Geometry: final body of the model. Coordinates: model frame, mm. A direction names the side the tool comes from. Round coordinates to 2 decimals unless told otherwise and drop trailing zeros. Loops run counter-clockwise (first coordinate to the right, second up) from the corner with the lowest first, then second, coordinate; pieces in that order, holes last. Notation, with made-up numbers: (61, 38.5) - (115, 38.5) arc R28 ccw to (115, 68.5) - close; hole circle Ø1 at (-38, 11). An arc over 180 degrees is marked (long way). Answer as CSV lines item,"result".
from build123d import *

# Parameters (mm, degrees)
BOSS_EXTRUDE1_DEPTH     = 10
SKETCH2_W               = 10
SKETCH2_H               = 2.000056303
BOSS_EXTRUDE2_DEPTH     = 5
CUT_EXTRUDE3_DEPTH      = 11
BOSS_EXTRUDE7_DEPTH     = 10
SKETCH10_R              = 42.5
CUT_EXTRUDE5_DEPTH      = 2
CUT_EXTRUDE5_DEPTH_BACK = 2


with BuildPart() as part:
    # Sketch1 → Boss-Extrude1 (new body)
    with BuildSketch(Plane.XY):
        with BuildLine():
            Line((-0.275264024, 0.618336289), (-0.275264024, 20.618336289))
            ThreePointArc((-0.275264024, 20.618336289), (-1.471073772, 23.494405264), (-4.353490365, 24.674832426))
            Line((-4.353490365, 24.674832426), (-4.353490365, 22.674776123))
            ThreePointArc((-4.353490365, 22.674776123), (-2.885297366, 22.080181828), (-2.275264024, 20.618336289))
            Line((-2.275264024, 20.618336289), (-2.275264024, 0.618336289))
            Line((-2.275264024, 0.618336289), (-1.040586258, -1.454212886))
            Line((-1.040586258, -1.454212886), (0.959413742, -1.454212886))
            Line((0.959413742, -1.454212886), (-0.275264024, 0.618336289))
        make_face()
    extrude(amount=BOSS_EXTRUDE1_DEPTH)

    # Sketch2 → Boss-Extrude2 (add)
    with BuildSketch(Plane.ZY.offset(4.353490365)):
        with Locations((5, 23.674804275)):
            Rectangle(SKETCH2_W, SKETCH2_H)
    extrude(amount=BOSS_EXTRUDE2_DEPTH)

    # Sketch7 → Cut-Extrude3 (cut, through all)
    with BuildSketch(Plane.XY.offset(10)):
        with BuildLine():
            Line((-9.353490365, 24.674832426), (-8.891740984, 22.674776123))
            ThreePointArc((-8.891740984, 22.674776123), (-9.122615674, 22.648471274), (-9.353490365, 22.674776123))
            Line((-9.353490365, 22.674776123), (-9.353490365, 24.674832426))
        make_face()
    extrude(amount=-CUT_EXTRUDE3_DEPTH, mode=Mode.SUBTRACT)

    # Sketch8 → Boss-Extrude7 (add, through all)
    with BuildSketch(Plane.XY.offset(10)):
        Polygon((-9.122615674, 23.674804274), (-50.533343428, 14.114384465), (-50.555838533, 14.211821471), (-9.14511078, 23.772241281), align=None)
    extrude(amount=-BOSS_EXTRUDE7_DEPTH)

    # Sketch10 → Cut-Extrude5 (cut, two sides)
    with BuildSketch(Plane(origin=(-5.673302165, 24.573771456, 0), x_dir=(0.974370065, 0.224951054, 0), z_dir=(-0.224951054, 0.974370065, 0))) as cut_extrude5_sk:
        with Locations((-45.063131443, -2.5)):
            Circle(SKETCH10_R)
    extrude(amount=CUT_EXTRUDE5_DEPTH, mode=Mode.SUBTRACT)
    extrude(cut_extrude5_sk.sketch, amount=-CUT_EXTRUDE5_DEPTH_BACK, mode=Mode.SUBTRACT)


solid = part.part
(1) Pin query (flat end, axial travel): P1, Ø1.5, axis at y = 10.5, z = 2, coming from the +X side; P2, Ø4, axis at x = -7.5, z = 5.5, coming from the -Y side; P3, Ø3, axis at y = 11, z = 5, coming from the -X side. Return the tip coordinate at first contact, or that it passes through.
Findings below:
P1,"x = -0.28"
P2,"y = 22.67"
P3,"x = -2.28"
(2) Section A-A (z = 8.25). Output: boundary loops of the cut face in (x, y), and give its area (3 significant figures).
Findings below:
outline,"(-8.73, 24.67) - (-8.27, 22.67) - (-4.35, 22.67) arc R2.06 cw to (-2.28, 20.62) - (-2.28, 0.62) - (-1.04, -1.45) - (0.96, -1.45) - (-0.28, 0.62) - (-0.28, 20.62) arc R4.06 ccw to (-4.35, 24.67) - close"
area,"62.1 mm2"
(3) Section C-C (y = 7.75). Output: boundary loops of the cut face in (x, z).
Findings below:
outline,"(-2.28, 0) - (-0.28, 0) - (-0.28, 10) - (-2.28, 10) - close"
(4) Draft query along Z for faces 1 (the face through (-2, 13, 10)), 2 (the face through (-1.44, 23.463, 4.93)), 3 (the face through (-8.187, 23.717, 5.088)), 4 (the face through (-2, 13, 0)). Return one class per face: pulls with the +Z half, pulls with the -Z half, needs draft (parallel to the pull), parting line crosses it, or undercut.
Findings below:
face 1,"pulls with the +Z half"
face 2,"needs draft"
face 3,"undercut"
face 4,"pulls with the -Z half"
(5) Section B-B (x = -7). Output: boundary loops of the cut face in (y, z), and give its area (3 significant figures).
Findings below:
outline,"(22.67, 0) - (24.67, 0) - (24.67, 10) - (22.67, 10) - close"
area,"20.0 mm2"
(6) Section D-D (z = 3.25). Output: boundary loops of the cut face in (x, y).
Findings below:
outline,"(-8.33, 24.67) - (-7.87, 22.67) - (-4.35, 22.67) arc R2.06 cw to (-2.28, 20.62) - (-2.28, 0.62) - (-1.04, -1.45) - (0.96, -1.45) - (-0.28, 0.62) - (-0.28, 20.62) arc R4.06 ccw to (-4.35, 24.67) - close"
(7) Material intervals for line 1 along X through (y, z) = (8.5, 2); line 2 along Y through (x, z) = (-5.5, 7.25); line 3 along Y through (x, z) = (-2.5, 2.5), sorted ascending.
Findings below:
line 1,"-2.28 to -0.28"
line 2,"22.67 to 24.67"
line 3,"21.55 to 24.24"
(8) Access query for faces 5 (the face through (-6, 22.675, 5)), 6 (the face through (-0.275, 10, 5)), 7 (the face through (0, -1.454, 5)). Directions: +Z, -Z, +X, -X, +Y, -Y. A direction counts if a zero-diameter tool reaches every point of the face in a straight line with its end or side. Return the directions, or none.
Findings below:
face 5,"+Z, -Z, -X, -Y"
face 6,"+Z, -Z, +X, +Y"
face 7,"+Z, -Z, +X, -X, -Y"
